```python
from build123d import *

# Parameters (mm, degrees)
EXTRUDE_1_DEPTH     = 4
CUT_EXTRUDE_1_REACH = 106.48
SKETCH_14_R         = 2
EXTRUDE_2_DEPTH     = 4
SKETCH_17_R         = 2.1
CUT_EXTRUDE_2_DEPTH = 10
EXTRUDE_3_DEPTH     = 4
FILLET_1_R          = 2


with BuildPart() as part:
    # 草图13 → 凸台-拉伸1 (new body)
    with BuildSketch(Plane.XY):
        Polygon((-30, -100), (0, -100), (0, 0), (0, 42.37433904), (-30, 22.517772204), align=None)
    extrude(amount=EXTRUDE_1_DEPTH)

    # 草图14 → 切除-拉伸1 (cut, up to next)
    with BuildSketch(Plane.XY.offset(4), mode=Mode.PRIVATE) as cut_extrude_1_sk1:
        with Locations((-22.5, -40)):
            Circle(SKETCH_14_R)
    cut_extrude_1_tool1 = extrude(cut_extrude_1_sk1.sketch, amount=-CUT_EXTRUDE_1_REACH, mode=Mode.PRIVATE) & part.part
    # 草图14 → 切除-拉伸1 (cut, up to next)
    with BuildSketch(Plane.XY.offset(4), mode=Mode.PRIVATE) as cut_extrude_1_sk2:
        with Locations((-7.5, -40)):
            Circle(SKETCH_14_R)
    cut_extrude_1_tool2 = extrude(cut_extrude_1_sk2.sketch, amount=-CUT_EXTRUDE_1_REACH, mode=Mode.PRIVATE) & part.part
    # 草图14 → 切除-拉伸1 (cut, up to next)
    with BuildSketch(Plane.XY.offset(4), mode=Mode.PRIVATE) as cut_extrude_1_sk3:
        with Locations((-7.5, -60)):
            Circle(SKETCH_14_R)
    cut_extrude_1_tool3 = extrude(cut_extrude_1_sk3.sketch, amount=-CUT_EXTRUDE_1_REACH, mode=Mode.PRIVATE) & part.part
    # 草图14 → 切除-拉伸1 (cut, up to next)
    with BuildSketch(Plane.XY.offset(4), mode=Mode.PRIVATE) as cut_extrude_1_sk4:
        with Locations((-7.5, -80)):
            Circle(SKETCH_14_R)
    cut_extrude_1_tool4 = extrude(cut_extrude_1_sk4.sketch, amount=-CUT_EXTRUDE_1_REACH, mode=Mode.PRIVATE) & part.part
    # 草图14 → 切除-拉伸1 (cut, up to next)
    with BuildSketch(Plane.XY.offset(4), mode=Mode.PRIVATE) as cut_extrude_1_sk5:
        with Locations((-22.5, -60)):
            Circle(SKETCH_14_R)
    cut_extrude_1_tool5 = extrude(cut_extrude_1_sk5.sketch, amount=-CUT_EXTRUDE_1_REACH, mode=Mode.PRIVATE) & part.part
    # 草图14 → 切除-拉伸1 (cut, up to next)
    with BuildSketch(Plane.XY.offset(4), mode=Mode.PRIVATE) as cut_extrude_1_sk6:
        with Locations((-22.5, -80)):
            Circle(SKETCH_14_R)
    cut_extrude_1_tool6 = extrude(cut_extrude_1_sk6.sketch, amount=-CUT_EXTRUDE_1_REACH, mode=Mode.PRIVATE) & part.part
    add(cut_extrude_1_tool1.solids().sort_by_distance((-22.5, -40, 4))[0], mode=Mode.SUBTRACT)
    add(cut_extrude_1_tool2.solids().sort_by_distance((-7.5, -40, 4))[0], mode=Mode.SUBTRACT)
    add(cut_extrude_1_tool3.solids().sort_by_distance((-7.5, -60, 4))[0], mode=Mode.SUBTRACT)
    add(cut_extrude_1_tool4.solids().sort_by_distance((-7.5, -80, 4))[0], mode=Mode.SUBTRACT)
    add(cut_extrude_1_tool5.solids().sort_by_distance((-22.5, -60, 4))[0], mode=Mode.SUBTRACT)
    add(cut_extrude_1_tool6.solids().sort_by_distance((-22.5, -80, 4))[0], mode=Mode.SUBTRACT)

    # 草图16 → 凸台-拉伸2 (add)
    with BuildSketch(Plane.XY.offset(4)):
        Polygon((-30, 22.517772204), (-55.160117038, 6.178601154), (-30, -32.564581559), align=None)
    extrude(amount=-EXTRUDE_2_DEPTH)

    # 草图17 → 切除-拉伸2 (cut)
    with BuildSketch(Plane.XY.offset(4)):
        with Locations((-3.429938262, 19.497880137)):
            Circle(SKETCH_17_R)
        with Locations((-25.627024556, 16.797998652)):
            Circle(SKETCH_17_R)
        with Locations((-36.785371145, -2.579599275)):
            Circle(SKETCH_17_R)
    extrude(amount=-CUT_EXTRUDE_2_DEPTH, mode=Mode.SUBTRACT)

    # 草图18 → 凸台-拉伸3 (add)
    with BuildSketch(Plane.XY.offset(4)):
        Polygon((0, 42.37433904), (19.317794486, 13.188335268), (0, -25.557166319), align=None)
    extrude(amount=-EXTRUDE_3_DEPTH)

    # 圆角1
    fillet_1_edges = [part.edges().sort_by_distance(p)[0] for p in [
        (-30, -32.564581559, 2),
        (-55.160117038, 6.178601154, 2),
        (0, -25.557166319, 2),
        (19.317794486, 13.188335268, 2),
        (0, 42.37433904, 2),
    ]]
    fillet(fillet_1_edges, radius=FILLET_1_R)


solid = part.part
```
Geometry: final body of the model. Coordinates: model frame, mm. A direction names the side the tool comes from. Coordinates: 2 decimals unless noted, no trailing zeros. Loops run counter-clockwise (first coordinate to the right, second up) from the corner with the lowest first, then second, coordinate; pieces in that order, holes last. Notation, with made-up numbers: (15, -24) -> (57, -24) arc R13 ccw to (57, -13) -> close; hole circle Ø5 at (-19.5, 84). An arc over 180 degrees is marked (long way). Use a Markdown table: item, result. Add a question column.
(1) Line query: line 1 along X through (y, z) = (-39.5, 1.8); line 2 along Y through (x, z) = (-23, 2.3); line 3 along Y through (x, z) = (-22.5, 1.65). Output: solid intervals per line, ascending.
(2) Mould query, pull axis X, two halves, no side actions, for faces 4 (the flat face through (-42.36, -13.53, 2.03)), 5 (the flat face through (9.636, -6.229, 2.028)), 6 (the cylindrical face through (-26.082, 14.748, 2.028)). Classes: pulls with the +X half, pulls with the -X half, needs draft (parallel to the pull), parting line crosses it, or undercut.
(3) Section query A-A, the plane y = -60. Return loops of the section in (x, z).
(4) Section query B-B, the plane z = 1.65. State how many separate pieces and enclosed holes the cut face has, plus the area to 3 significant figures.
(5) Pin query (flat end, axial travel): pin 1 Ø1.2 at (y, z) = (-58.5, 3) entering from +X; pin 2 Ø2 at (x, z) = (-42.5, 2.5) entering from +Y. Return the tip coordinate at first contact, or that it passes through.
(6) Section query C-C, the plane x = -7.5. Return loops of the section in (y, z), plus the area to 3 significant figures.
(7) Access query for faces 1 (the flat face through (-30, -66, 2)), 2 (the flat face through (0, -64, 2)), 3 (the cylindrical face through (-54.345, 6.028, 1.972)). Directions: +Z, -Z, +X, -X, +Y, -Y. A direction counts if a zero-diameter tool reaches every point of the face in a straight line with its end or side. Return the directions, or none.
(8) Section query D-D, the plane x = -45. Return loops of the section in (y, z), plus the area to 3 significant figures.
Answer:
| question | item | result |
|---|---|---|
| 1 | line 1 | x = -30 to -24.44, -20.56 to -9.44, -5.56 to 0 |
| 1 | line 2 | y = -100 to -81.94, -78.06 to -61.94, -58.06 to -41.94, -38.06 to 27.15 |
| 1 | line 3 | y = -100 to -82, -78 to -62, -58 to -42, -38 to 27.48 |
| 2 | face 4 | pulls with the -X half |
| 2 | face 5 | pulls with the +X half |
| 2 | face 6 | undercut |
| 3 | outline | (-30, 0) -> (-24.5, 0) -> (-24.5, 4) -> (-30, 4) -> close; (-20.5, 0) -> (-9.5, 0) -> (-9.5, 4) -> (-20.5, 4) -> close; (-5.5, 0) -> (0, 0) -> (0, 4) -> (-5.5, 4) -> close |
| 4 | separate pieces | 1 |
| 4 | enclosed holes | 9 |
| 4 | area | 5,200 mm^2 |
| 5 | pin 1 | stops at x = 0 |
| 5 | pin 2 | stops at y = 15.05 |
| 6 | outline | (-100, 0) -> (-82, 0) -> (-82, 4) -> (-100, 4) -> close; (-78, 0) -> (-62, 0) -> (-62, 4) -> (-78, 4) -> close; (-58, 0) -> (-42, 0) -> (-42, 4) -> (-58, 4) -> close; (-38, 0) -> (37.41, 0) -> (37.41, 4) -> (-38, 4) -> close |
| 6 | area | 502 mm^2 |
| 7 | face 1 | +Z, -Z, -X, -Y |
| 7 | face 2 | +Z, -Z, +X, -Y |
| 7 | face 3 | +Z, -Z, -X |
| 8 | outline | (-9.47, 0) -> (12.78, 0) -> (12.78, 4) -> (-9.47, 4) -> close |
| 8 | area | 89.0 mm^2 |
